```python
from build123d import *

# Parameters (mm, degrees)
SKETCH_1_W          = 36.9
SKETCH_1_H          = 39
EXTRUDE_1_DEPTH     = 7
SKETCH_2_W          = 24
SKETCH_2_H          = 37.5
EXTRUDE_2_DEPTH     = 5
SKETCH_4_W          = 39.5
SKETCH_4_H          = 10
EXTRUDE_3_DEPTH     = 3
EXTRUDE_4_DEPTH     = 10
CUT_EXTRUDE_3_DEPTH = 10
CUT_EXTRUDE_START   = 0.2
CUT_EXTRUDE_4_DEPTH = 0.2
CUT_EXTRUDE_START_2 = -10
CUT_EXTRUDE_5_DEPTH = 0.2
FILLET_1_R          = 5
FILLET_2_R          = 1
MIRROR_START        = 20.8
MIRROR_4_DEPTH      = 10.4
MIRROR_START_2      = 21
MIRROR_4_2_DEPTH    = 10
FILLET_3_R          = 1
SKETCH_7_W          = 3
SKETCH_7_H          = 37.5
EXTRUDE_5_DEPTH     = 2
FILLET_4_R          = 3
SKETCH_8_R          = 1.95
CUT_EXTRUDE_6_DEPTH = 65.569807186


# Read off the part's stored shape, not the designer's step: 鏡射4
with BuildPart() as part:
    # 草圖1 → 填料-伸長1 (new body)
    with BuildSketch(Plane.XY):
        with Locations((18.45, 19.5)):
            Rectangle(SKETCH_1_W, SKETCH_1_H)
    extrude(amount=EXTRUDE_1_DEPTH)

    # 草圖2 → 填料-伸長2 (add)
    with BuildSketch(Plane.XZ):
        with Locations((18.45, 18.75)):
            Rectangle(SKETCH_2_W, SKETCH_2_H)
    extrude(amount=EXTRUDE_2_DEPTH)

    # 草圖4 → 填料-伸長3 (add)
    with BuildSketch(Plane(origin=(36.9, 0, 0), x_dir=(0, 0, -1), z_dir=(1, 0, 0))):
        with Locations((-19.75, 26)):
            Rectangle(SKETCH_4_W, SKETCH_4_H)
    extrude(amount=EXTRUDE_3_DEPTH)

    # 草圖5 → 填料-伸長4 (add)
    with BuildSketch(Plane(origin=(0, 31, 0), x_dir=(1, 0, 0), z_dir=(0, 1, 0))):
        Polygon((36.9, -39.5), (35.069872981, -37.669872981), (36.9, -34.5), align=None)
    extrude(amount=-EXTRUDE_4_DEPTH)

    # 草圖6 → 除料-伸長3 (cut)
    with BuildSketch(Plane(origin=(0, 31, 0), x_dir=(1, 0, 0), z_dir=(0, 1, 0))):
        with BuildLine():
            Line((36.398110453, -7), (36.899055226, -7))
            Line((36.899055226, -7), (37.4, -6.1323382))
            Line((37.4, -6.1323382), (37.4, -5))
            ThreePointArc((37.4, -5), (36.899055226, -4.499055226), (36.398110453, -5))
            Line((36.398110453, -5), (36.398110453, -7))
        make_face()
    extrude(amount=-CUT_EXTRUDE_3_DEPTH, mode=Mode.SUBTRACT)

    # 草圖6<2> → 除料-伸長4 (cut)
    with BuildSketch(Plane(origin=(0, 31, 0), x_dir=(1, 0, 0), z_dir=(0, 1, 0)).offset(CUT_EXTRUDE_START)):
        with BuildLine():
            Line((36.398110453, -7), (36.899055226, -7))
            Line((36.899055226, -7), (37.4, -6.1323382))
            Line((37.4, -6.1323382), (37.4, -5))
            ThreePointArc((37.4, -5), (36.899055226, -4.499055226), (36.398110453, -5))
            Line((36.398110453, -5), (36.398110453, -7))
        make_face()
    extrude(amount=-CUT_EXTRUDE_4_DEPTH, mode=Mode.SUBTRACT)

    # 草圖6<3> → 除料-伸長5 (cut)
    with BuildSketch(Plane(origin=(0, 31, 0), x_dir=(1, 0, 0), z_dir=(0, 1, 0)).offset(CUT_EXTRUDE_START_2)):
        with BuildLine():
            Line((36.398110453, -7), (36.899055226, -7))
            Line((36.899055226, -7), (37.4, -6.1323382))
            Line((37.4, -6.1323382), (37.4, -5))
            ThreePointArc((37.4, -5), (36.899055226, -4.499055226), (36.398110453, -5))
            Line((36.398110453, -5), (36.398110453, -7))
        make_face()
    extrude(amount=-CUT_EXTRUDE_5_DEPTH, mode=Mode.SUBTRACT)

    # 圓角1
    fillet_1_edges = [part.edges().sort_by_distance(p)[0] for p in [
        (6.45, 0, 3.5),
        (30.45, 0, 3.5),
    ]]
    fillet(fillet_1_edges, radius=FILLET_1_R - 0.0001)  # a hair under: the kernel refuses the full size

    # 圓角2
    fillet_2_edges = [part.edges().sort_by_distance(p)[0] for p in [
        (36.9, 26, 39.5),
    ]]
    fillet(fillet_2_edges, radius=FILLET_2_R)

    # 鏡射4 outline → 鏡射4 (cut)
    with BuildSketch(Plane(origin=(0, 0, 0), x_dir=(1, 0, 0), z_dir=(0, 1, 0)).offset(MIRROR_START)):
        with BuildLine():
            Line((0, -4.499056117), (0, -6.998363603))
            Line((0, -6.998363603), (0.000944774, -7))
            Line((0.000944774, -7), (0.501889547, -7))
            Line((0.501889547, -7), (0.501889547, -5))
            ThreePointArc((0.501889547, -5), (0.354832035, -4.645444683), (0, -4.499056117))
        make_face()
    extrude(amount=MIRROR_4_DEPTH, mode=Mode.SUBTRACT)

    # Mirror 4 2 outline → Mirror 4 2 (add)
    with BuildSketch(Plane(origin=(0, 0, 0), x_dir=(1, 0, 0), z_dir=(0, 1, 0)).offset(MIRROR_START_2)):
        with BuildLine():
            Line((0, -34.5), (0, -6.998363603))
            Line((0, -6.998363603), (-0.5, -6.1323382))
            Line((-0.5, -6.1323382), (-0.5, -5))
            ThreePointArc((-0.5, -5), (-0.353610544, -4.646112739), (0, -4.499056117))
            Line((0, -4.499056117), (0, 0))
            Line((0, 0), (-3, 0))
            Line((-3, 0), (-3, -39.5))
            Line((-3, -39.5), (0, -39.5))
            Line((0, -39.5), (1.830127019, -37.669872981))
            Line((1.830127019, -37.669872981), (0, -34.5))
        make_face()
    extrude(amount=MIRROR_4_2_DEPTH)

    # 圓角3
    fillet_3_edges = [part.edges().sort_by_distance(p)[0] for p in [
        (0, 26, 39.5),
    ]]
    fillet(fillet_3_edges, radius=FILLET_3_R)

    # 草圖7 → 填料-伸長5 (add)
    with BuildSketch(Plane.XZ.offset(5)):
        with Locations((13.45, 18.75)):
            Rectangle(SKETCH_7_W, SKETCH_7_H)
        with Locations((23.45, 18.75)):
            Rectangle(SKETCH_7_W, SKETCH_7_H)
    extrude(amount=EXTRUDE_5_DEPTH)

    # 圓角4
    fillet_4_edges = [part.edges().sort_by_distance(p)[0] for p in [
        (13.45, -7, 37.5),
    ]]
    fillet(fillet_4_edges, radius=FILLET_4_R)

    # 草圖8 → 除料-伸長6 (cut, through all)
    with BuildSketch(Plane.XY.offset(7)):
        with Locations((18.45, 29)):
            Circle(SKETCH_8_R)
        with Locations((18.45, 14)):
            Circle(SKETCH_8_R)
    extrude(amount=-CUT_EXTRUDE_6_DEPTH, mode=Mode.SUBTRACT)


solid = part.part
```
Here's how the part is built. I have some questions about the finished solid (model axes, mm). A direction names the side the tool comes from. Give positions to 0.01 mm unless a question says otherwise; leave off trailing zeros. Order: outer loops, then holes, each group sorted by start corner. A loop starts at its lowest first (then second) coordinate and runs counter-clockwise, first axis right, second up. Notation, with made-up numbers: M 56,-32.5 L 92,-32.5 A24 cw 92,1.5 Z; hole C 20.5,4.25 d7. An arc over 180 degrees is marked long. Use a Markdown table: item, result. Add a question column.
1. On a 3-axis mill with a long thin cutter (end or side, diameter ignored), from which of +Z, -Z, +X, -X, +Y, -Y can I reach the whole of each face in a straight line? I mean faces 4 (the flat face through (6.45, -2, 23)), 5 (the flat face through (36.9, 26, 21)), 6 (the flat face through (21.95, -6, 18)), 7 (the flat face through (1.1, 25.9, 38.4)), 8 (the flat face through (11.95, -6, 18)). Say none if no direction works.
2. Suppose I cut it at D-D (x = 14). List the corners of the cut face in (y, z) for me, and give its area (3 significant figures).
3. For pin 1 Ø1.5 at (y, z) = (-1.5, 7) entering from -X; pin 2 Ø2 at (y, z) = (9, 3.5) entering from -X; pin 3 Ø4 at (x, y) = (26, 31) entering from +Z, each with a flat end and sliding along its axis, tell me the tip position at first contact or that it passes through.
4. If we mould it in two halves opening along Z, with no side actions, what happens to faces 1 (the flat face through (35.97, 26.07, 36.11)), 2 (the flat face through (30.45, -2, 23)), 3 (the cylindrical face through (18.618, -4.745, 37.406))? For each: +Z half, -Z half, draft (parallel to the pull), parting line (faces both ways), or undercut.
5. Suppose I cut it at A-A (y = 14). List the corners of the cut face in (x, z) for me.
6. I need wall thicknesses on probe 1 along Y at (x, z) = (18.45, 2.5); probe 2 along Z at (x, y) = (17.5, 33); probe 3 along Y at (x, z) = (25, 24). Which ranges of each line are inside material? Lowest first, please. Write a range as from..to.
7. Suppose I cut it at B-B (z = 23). List the corners of the cut face in (x, y) for me, and give its area (3 significant figures).
8. Suppose I cut it at C-C (x = 18.45). List the corners of the cut face in (y, z) for me.
Results list:
| question | item | result |
|---|---|---|
| 1 | face 4 | +Z, -X, +Y, -Y |
| 1 | face 5 | +Y, -Y |
| 1 | face 6 | +Z, -Z, -Y |
| 1 | face 7 | +Z, +Y, -Y |
| 1 | face 8 | +Z, -Z, -X, -Y |
| 2 | outline | M -7,0 L 39,0 L 39,7 L 0,7 L 0,37.5 L -4,37.5 A3 ccw -7,34.5 Z |
| 2 | area | 534 mm² |
| 3 | pin 1 | stops at x = 4.08 |
| 3 | pin 2 | stops at x = 0 |
| 3 | pin 3 | stops at z = 7 |
| 4 | face 1 | undercut |
| 4 | face 2 | draft |
| 4 | face 3 | +Z half |
| 5 | outline | M 0,0 L 16.5,0 L 16.5,7 L 0,7 Z; M 20.4,0 L 36.9,0 L 36.9,7 L 20.4,7 Z |
| 6 | probe 1 | y = -5..12.05, 15.95..27.05, 30.95..39 |
| 6 | probe 2 | z = 0..7 |
| 6 | probe 3 | y = -5..0 |
| 7 | outline | M -3,21 L 0,21 L 0,31 L -3,31 Z; M 6.45,-5 L 11.95,-5 L 11.95,-7 L 14.95,-7 L 14.95,-5 L 21.95,-5 L 21.95,-7 L 24.95,-7 L 24.95,-5 L 30.45,-5 L 30.45,0 L 6.45,0 Z; M 36.9,21 L 39.9,21 L 39.9,31 L 36.9,31 Z |
| 7 | area | 192 mm² |
| 8 | outline | M -5,0 L 12.05,0 L 12.05,7 L 0,7 L 0,37.5 L -4,37.5 A3 ccw -5,37.33 Z; M 15.95,0 L 27.05,0 L 27.05,7 L 15.95,7 Z; M 30.95,0 L 39,0 L 39,7 L 30.95,7 Z |
